The model under review builds one solid part; all positions refer to its coordinate system, in mm. A direction names the side the tool comes from. Coordinates: 2 decimals unless noted, no trailing zeros. Loops run counter-clockwise (first coordinate to the right, second up) from the corner with the lowest first, then second, coordinate; pieces in that order, holes last. Notation, with made-up numbers: M 45.25,35.5 L 67.25,35.5 A32 cw 67.25,66.5 Z; hole C 23,-37 d8. An arc over 180 degrees is marked long. Use one line per item in the form item = value.
Autodesk Inventor part; units mm, degrees
ref_plane "YZ Plane" through (0, 0, 0) normal (1, 0, 0) x (0, 1, 0)
ref_plane "XZ Plane" through (0, 0, 0) normal (0, 1, 0) x (-1, 0, 0)
ref_plane "XY Plane" through (0, 0, 0) normal (0, 0, 1) x (1, 0, 0)
sketch "Sketch1" plane through (0, 0, 0) normal (0, 0, 1) x (1, 0, 0)
  line L0 (-67, 120) -> (67, 120)
  line L1 (67, 120) -> (67, 0)
  line L2 (67, 0) -> (-67, 0)
  line L3 (-67, 0) -> (-67, 120)
  line L4 (-45.5, 120) -> (45.5, 120)
  line L5 (45.5, 120) -> (45.5, 30)
  line L6 (45.5, 30) -> (-45.5, 30)
  line L7 (-45.5, 30) -> (-45.5, 120)
  point P0 (0, 0)
  point P1 (0, 0)
  point P2 (0, 30)
  dimension "d0" = 134
  dimension "d1" = 120
  dimension "d2" = 91
  dimension "d3" = 90
extrude "Extrusion1" add sketch "Sketch1" along normal mid plane 50 contours L0 L7 L6 L5 L1 L2 L3
sketch "Sketch2" plane through (-45.5, 30, -25) normal (0, 1, 0) x (1, 0, 0)
  point P0 (45.5, -25)
  point P1 (45.5, -25)
hole "Hole1" at (0, 30, 0) direction (0, -1, 0) diameter 9 end through all counterbore diameter 15 counterbore depth 15
sketch "Sketch3" plane through (67, 0, 25) normal (1, 0, 0) x (0, 0, -1)
  line L0 (50, 120) -> (0, 120)
  circle A0 centre (25, 126) radius 14
  point P0 (25, 0)
  point P1 (12.3509, 120)
  point P2 (37.6491, 120)
  dimension "d16" = 28
  dimension "d17" = 6
extrude "Extrusion2" cut sketch "Sketch3" along normal through all both and the other way through all contours A0 L0 picked at (25, 117.3333)
fillet "Fillet1" radius 15 4 edges at (67, 0, 0) (-67, 0, 0) (-45.5, 30, 0) (45.5, 30, 0)
fillet "Fillet2" radius 3 12 edges at (-45.5, 120, -18.8246) (-67, 120, -18.8246) (-67, 120, 18.8246) (-45.5, 120, 18.8246) (45.5, 120, -18.8246) (67, 120, -18.8246) (67, 120, 18.8246) (45.5, 120, 18.8246) (45.5, 112, 0) (67, 112, 0) (-45.5, 112, 0) (-67, 112, 0)
chamfer "Chamfer1" distance 0.6 angle 45 28 edges at (-45.5, 81, 25) (-46.3787, 119.1213, 25) (-56.25, 120, 25) (-66.1213, 119.1213, 25) (-67, 66, 25) (-62.6066, 4.3934, 25) (0, 0, 25) (62.6066, 4.3934, 25) (67, 66, 25) (66.1213, 119.1213, 25) (56.25, 120, 25) (46.3787, 119.1213, 25) (45.5, 81, 25) (0, 30, 25) (67, 66, -25) (62.6066, 4.3934, -25) (0, 0, -25) (-62.6066, 4.3934, -25) (-67, 66, -25) (-66.1213, 119.1213, -25) (-56.25, 120, -25) (-46.3787, 119.1213, -25) (-45.5, 81, -25) (0, 30, -25) (45.5, 81, -25) (46.3787, 119.1213, -25) (56.25, 120, -25) (66.1213, 119.1213, -25)
sketch "Sketch4" plane through (48.5, 120, -12.6491) normal (0, 1, 0) x (1, 0, 0)
  line L0 (7.75, -31.6491) -> (7.75, 6.3509) construction
  line L1 (15.5, -37.0491) -> (0, -37.0491)
  point P0 (-48.5, -12.6491)
  point P1 (7.75, -37.0491)
  point P2 (7.75, -12.6491)
  dimension "d30" = 38
hole "Hole2" at (56.25, 120, -19) at (56.25, 120, 19) direction (0, -1, 0) diameter 4.8 depth 10 tip angle 118 counterbore diameter 5.2 counterbore depth 1
mirror "Mirror1" about plane through (0, 0, 0) normal (1, 0, 0) of "Hole2"
chamfer "Chamfer2" distance 0.5 angle 45 4 edges at (0, 30, -7.5) (0, 0, -4.5) (0, 15, -4.5) (0, 15, -7.5)
equation "\"d0\" = width"
equation "\"d1\" = hight"
equation "\"d2\" = gap"
equation "\"d3\" = verticalgap"
equation "\"width\" = 134"
equation "\"hight\" = 120"
equation "\"gap\" = 91"
equation "\"verticalgap\" = 90"
properties part number "pld-support" material "ABS Plastic"
1. Wall thickness on line 1 along X through (y, z) = (112.25, 19); line 2 along X through (y, z) = (20, 0); line 3 along Z through (x, y) = (56.25, 119.55): over which ranges is each line inside the solid? List them lowest first. Write a range as from..to.
Response values:
line_1 = -67..-58.65, -53.85..-45.5, 45.5..53.85, 58.65..67
line_2 = -67..-7.5, 7.5..67
line_3 = -24.85..-21.6, -16.4..-12.43, 12.43..16.4, 21.6..24.85
2. Add section B-B (y = 94). State the section outline as (x, z) points.
Response values:
outline = M -67,-24.4 L -66.4,-25 L -46.1,-25 L -45.5,-24.4 L -45.5,24.4 L -46.1,25 L -66.4,25 L -67,24.4 Z; M 45.5,-24.4 L 46.1,-25 L 66.4,-25 L 67,-24.4 L 67,24.4 L 66.4,25 L 46.1,25 L 45.5,24.4 Z
3. Add section D-D (x = -19). State the section outline as (y, z) points.
Response values:
outline = M 0,-24.4 L 0.6,-25 L 29.4,-25 L 30,-24.4 L 30,24.4 L 29.4,25 L 0.6,25 L 0,24.4 Z
4. Add section A-A (x = 0). State the section outline as (y, z) points.
Response values:
outline = M 0,-24.4 L 0.6,-25 L 29.4,-25 L 30,-24.4 L 30,-8 L 29.5,-7.5 L 15.5,-7.5 L 15,-7 L 15,-5 L 14.5,-4.5 L 0.5,-4.5 L 0,-5 Z; M 0,5 L 0.5,4.5 L 14.5,4.5 L 15,5 L 15,7 L 15.5,7.5 L 29.5,7.5 L 30,8 L 30,24.4 L 29.4,25 L 0.6,25 L 0,24.4 Z
5. Insertion check: P1, Ø2.5, axis at x = -57, z = -18, coming from the +Y side; P2, Ø5.5, axis at x = 56.25, z = -19, coming from the -Y side; P3, Ø7, axis at x = -56.25, z = -19, coming from the -Y side; P4, Ø6, axis at x = 56.25, z = 19, coming from the +Y side. Each pin has a flat end and moves straight along its axis. Give the tip position at first contact, or say it passes through.
Response values:
P1 = 119
P2 = 0.08
P3 = 0.02
P4 = 120
6. The part is to be moulded in two halves that separate along X. For faces 5 (the face through (-54.12, 114.44, 20.11)), 6 (the face through (-66.1, 119.14, -18.44)), 7 (the face through (65.838, 118.798, -24.829)), 8 (the face through (56, 120, -16)), say which applies: pulls with the +X half, pulls with the -X half, needs draft (parallel to the pull), parting line crosses it, or undercut.
Response values:
face_5 = undercut
face_6 = pulls with the -X half
face_7 = pulls with the +X half
face_8 = needs draft
7. Machinability: for faces 1 (the face through (58.38, 114.44, -17.89)), 2 (the face through (46.702, 118.838, -24.829)), 3 (the face through (62.189, 4.584, -24.829)), 4 (the face through (46.36, 119.1, 18.44)), which of the approach directions +Z, -Z, +X, -X, +Y, -Y give a long, thin tool a straight path to every point of the face, cutting with its end or side? Answer none if there is none.
Response values:
face_1 = +Y
face_2 = -Z, +Y
face_3 = -Z, +X, -Y
face_4 = +Z, -Z, +Y
